Check sheet for the modelled part. Datum: model origin and axes. Units: mm. Face numbers are marked on the shaded views. A direction names the side the tool comes from. Round coordinates to 2 decimals unless told otherwise and drop trailing zeros. Write each loop counter-clockwise with the first axis right and the second up, starting at its lowest first coordinate (ties: lowest second). Pieces come first, ordered by that corner, then holes. Notation, with made-up numbers: (84, 74) -> (107, 74) arc R8 ccw to (107, 78) -> close; hole circle Ø9 at (-21, 19). An arc over 180 degrees is marked (long way). Put each result on its own line as item: value. Start each with the question number.
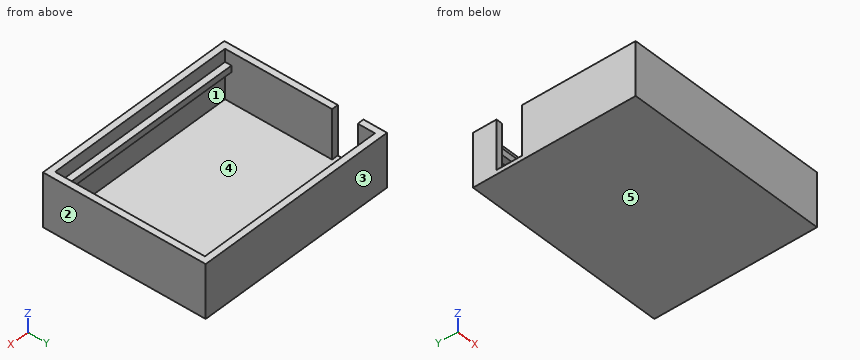
from build123d import *

# Parameters (mm, degrees)
PAD_DEPTH    = 25
SKETCH001_W  = 96
SKETCH001_H  = 76
PAD001_DEPTH = 2
SKETCH002_W  = 96
SKETCH002_H  = 3
PAD002_DEPTH = 3
SKETCH003_W  = 96
SKETCH003_H  = 3
PAD003_DEPTH = 3


with BuildPart() as part:
    # Sketch → Pad (new body)
    with BuildSketch(Plane.XY):
        Polygon((0, 0), (96, 0), (96, 76), (0, 76), (0, 65), (3, 65), (3, 73), (93, 73), (93, 3), (3, 3), (3, 53), (0, 53), align=None)
    extrude(amount=PAD_DEPTH)

    # Sketch001 → Pad001 (join)
    with BuildSketch(Plane.XY):
        with Locations((48, 38)):
            Rectangle(SKETCH001_W, SKETCH001_H)
    extrude(amount=PAD001_DEPTH)

    # Sketch002 → Pad002 (join)
    with BuildSketch(Plane.XY.offset(16)):
        with Locations((48, 4.5)):
            Rectangle(SKETCH002_W, SKETCH002_H)
    extrude(amount=PAD002_DEPTH)

    # Sketch003 → Pad003 (join)
    with BuildSketch(Plane.XY.offset(17)):
        with Locations((48, 71.5)):
            Rectangle(SKETCH003_W, SKETCH003_H)
    extrude(amount=PAD003_DEPTH)


solid = part.part
1. Section check B-B, the plane z = 10.75. Enter the section's corners in (x, y), then the cut area to 3 significant figures.
2. Section check D-D, the plane y = 9. Enter the section's corners in (x, z).
3. Gauge pin test, flat ends, axial feed: P1, Ø3, axis at x = 76.5, y = 55.5, coming from the +Z side; P2, Ø6, axis at y = 57.5, z = 17.5, coming from the -X side; P3, Ø2.5, axis at x = 68.5, y = 4.5, coming from the +Z side. Record the tip position at first contact, or that the pin passes through.
4. Access from +Z, -Z, +X, -X, +Y, -Y to the whole of each face (thin tool, end or side, straight path). Record for the marked faces 1 and 2.
5. Section check A-A, the plane y = 60.5. Enter the section's corners in (x, z), then the cut area to 3 significant figures.
6. Section check C-C, the plane x = 19. Enter the section's corners in (y, z), then the cut area to 3 significant figures.
7. Material ranges on L1, parallel to Y at x = 31, z = 6; L2, parallel to X at y = 19, z = 7.75; L3, parallel to Y at x = 70, z = 18, recorded low to high. Write a range as [from, to].
8. Draft check along Y on the marked faces 3, 4 and 5. Enter one of: released by +Y, released by -Y, zero draft, split by the parting line, or undercut.
Reply:
1. outline: (0, 0) -> (96, 0) -> (96, 76) -> (0, 76) -> (0, 65) -> (3, 65) -> (3, 73) -> (93, 73) -> (93, 3) -> (3, 3) -> (3, 53) -> (0, 53) -> close
1. area: 960 mm2
2. outline: (0, 0) -> (96, 0) -> (96, 25) -> (93, 25) -> (93, 2) -> (3, 2) -> (3, 25) -> (0, 25) -> close
3. P1: stops at z = 2
3. P2: stops at x = 93
3. P3: stops at z = 19
4. face 1: none
4. face 2: +Z, -Z, +X, +Y, -Y
5. outline: (0, 0) -> (96, 0) -> (96, 25) -> (93, 25) -> (93, 2) -> (0, 2) -> close
5. area: 261 mm2
6. outline: (0, 0) -> (76, 0) -> (76, 25) -> (73, 25) -> (73, 20) -> (70, 20) -> (70, 17) -> (73, 17) -> (73, 2) -> (3, 2) -> (3, 16) -> (6, 16) -> (6, 19) -> (3, 19) -> (3, 25) -> (0, 25) -> close
6. area: 308 mm2
7. L1: y = [0, 3], [73, 76]
7. L2: x = [0, 3], [93, 96]
7. L3: y = [0, 6], [70, 76]
8. face 3: released by +Y
8. face 4: undercut
8. face 5: zero draft
